```python
from build123d import *

# Parameters (mm, degrees)
SKETCH1_R               = 90
BOSS_EXTRUDE1_DEPTH     = 2
CUT_EXTRUDE2_DEPTH      = 128.294933128
SKETCH9_R               = 1.75
CUT_EXTRUDE7_DEPTH      = 128.294933128
CUT_EXTRUDE8_DEPTH      = 128.294933128
CUT_EXTRUDE8_DEPTH_BACK = 128.294933128
CHAMFER3_SIZE           = 1
SKETCH17_R              = 6
CUT_EXTRUDE9_DEPTH      = 99.491613961


with BuildPart() as part:
    # Sketch1 → Boss-Extrude1 (new body)
    with BuildSketch(Plane(origin=(0, 0, 0), x_dir=(1, 0, 0), z_dir=(0, 1, 0))):
        with Locations(Location((0, 0, 0), (0, 0, 270))):
            Circle(SKETCH1_R)
    extrude(amount=BOSS_EXTRUDE1_DEPTH)

    # Sketch4 → Cut-Extrude2 (cut, through all)
    with BuildSketch(Plane(origin=(0, 2, 0), x_dir=(1, 0, 0), z_dir=(0, 1, 0))):
        with BuildLine():
            Line((-42.5, 79.333158263), (-42.5, 69.333158263))
            ThreePointArc((-42.5, 69.333158263), (0, 55), (42.5, 69.333158263))
            Line((42.5, 69.333158263), (42.5, 79.333158263))
            Line((42.5, 79.333158263), (42.5, 105.809765059))
            Line((42.5, 105.809765059), (-42.5, 105.809765059))
            Line((-42.5, 105.809765059), (-42.5, 79.333158263))
        make_face()
    extrude(amount=-CUT_EXTRUDE2_DEPTH, mode=Mode.SUBTRACT)

    # Sketch9 → Cut-Extrude7 (cut, through all)
    with BuildSketch(Plane(origin=(0, 2, 0), x_dir=(1, 0, 0), z_dir=(0, 1, 0))):
        with Locations(Location((-49.706440821, 70.180266036, 0), (0, 0, 270))):
            Circle(SKETCH9_R)
    cut_extrude7 = extrude(amount=-CUT_EXTRUDE7_DEPTH, mode=Mode.SUBTRACT)

    # Mirror1: Cut-Extrude7 across plane
    add(cut_extrude7.mirror(Plane(origin=(0, 0, 0), x_dir=(0, 0, 1), z_dir=(1, 0, 0))), mode=Mode.SUBTRACT)

    # Sketch10 → Cut-Extrude8 (cut, two sides)
    with BuildSketch(Plane.XZ) as cut_extrude8_sk:
        Polygon((349.590781265, -403.844847198), (57.81736756, -68.972110366), (50, -60), (25, -35), (-25, -35), (-50, -60), (-57.81736756, -68.972110366), (-349.590781265, -403.844847198), (-349.590781265, 484.460223862), (349.590781265, 484.460223862), align=None)
    extrude(amount=CUT_EXTRUDE8_DEPTH, mode=Mode.SUBTRACT)
    extrude(cut_extrude8_sk.sketch, amount=-CUT_EXTRUDE8_DEPTH_BACK, mode=Mode.SUBTRACT)

    # Sketch15 for Loft1 → Loft1 section 0
    with BuildSketch(Plane(origin=(0, -6, 0), x_dir=(1, 0, 0), z_dir=(0, 1, 0))):
        with BuildLine():
            Line((-42.5, 69.333158263), (-42.5, 79.333158263))
            # circular arc as an exact rational Bezier (weights 1, cos(half-angle), 1)
            Bezier((-42.5, 79.333158263), (0, 57.45059928), (42.5, 79.333158263), weights=[1, 0.889071458, 1])
            Line((42.5, 79.333158263), (42.5, 69.333158263))
            Bezier((42.5, 69.333158263), (0, 36.987960736), (-42.5, 69.333158263), weights=[1, 0.795754331, 1])
        make_face()
    # Sketch16 for Loft1 → Loft1 section 1
    with BuildSketch(Plane.XZ):
        with BuildLine():
            Line((-45.948502669, -63.851980058), (-42.5, -69.333158263))
            Bezier((-42.5, -69.333158263), (0, -36.987960736), (42.5, -69.333158263), weights=[1, 0.795754331, 1])
            Line((42.5, -69.333158263), (44.152042302, -63.851980058))
            Bezier((44.152042302, -63.851980058), (-0.898230184, -19.650095816), (-45.948502669, -63.851980058), weights=[1, 0.713795953, 1])
        make_face()
    loft()

    # Chamfer3
    chamfer3_edges = [part.edges().sort_by_distance(p)[0] for p in [
        (0, 2, -55),
    ]]
    chamfer(chamfer3_edges, length=CHAMFER3_SIZE)

    # Sketch17 → Cut-Extrude9 (cut, through all)
    with BuildSketch(Plane(origin=(0, 2, 0), x_dir=(1, 0, 0), z_dir=(0, 1, 0))):
        with Locations(Location((2.697741472, 47.316027374, 0), (0, 0, 270))):
            Circle(SKETCH17_R)
        with Locations(Location((27.628576658, 52.274065286, 0), (0, 0, 270))):
            Circle(SKETCH17_R)
        with Locations(Location((-29.151926102, 52.274065286, 0), (0, 0, 270))):
            Circle(SKETCH17_R)
    extrude(amount=-CUT_EXTRUDE9_DEPTH, mode=Mode.SUBTRACT)


solid = part.part
```
Design review of the part built by this model. Coordinates are the model's own, in mm. A direction names the side the tool comes from. Give positions to 0.01 mm unless a question says otherwise; leave off trailing zeros. Order: outer loops, then holes, each group sorted by start corner. A loop starts at its lowest first (then second) coordinate and runs counter-clockwise, first axis right, second up. Notation, with made-up numbers: (8.25, 82.25) - (28.25, 82.25) arc R20 ccw to (28.25, 115.25) - close; hole circle Ø9 at (-27.5, 38.25). An arc over 180 degrees is marked (long way). Use a Markdown table: item, result. Add a question column.
(1) Mouldability with a two-part tool opening along Z and no side actions: class faces 1 (the face through (0, 1, -35)), 2 (the face through (-0.6, 1.2, -54.8)), 3 (the face through (-28.89, -0.43, -58.27)) as +Z half, -Z half, draft (parallel to the pull), parting line (faces both ways), or undercut.
(2) Add section A-A on z = -57. Give the number of separate pieces and of enclosed holes in the cut face, then the cut area to 3 significant figures.
(3) Clearance check with flat-ended pins moving along their axes: P1, Ø5, axis at x = -25, z = -55, coming from the -Y side; P2, Ø2, axis at x = -14.5, y = -5, coming from the +Z side; P3, Ø12, axis at x = 46, z = -53.5, coming from the -Y side; P4, Ø15.5, axis at x = 2.7, z = -47.32, coming from the +Y side. State where each tip first meets the part, or that it passes through.
(4) Add section B-B on z = -40. Give the boundary of the cut face in (x, y).
(5) Machinability: for faces 4 (the face through (2.96, -0.64, -53.31)), 5 (the face through (-0.639, 0.507, -55.003)), which of the approach directions +Z, -Z, +X, -X, +Y, -Y give a long, thin tool a straight path to every point of the face, cutting with its end or side? Answer none if there is none.
(6) Wall thickness on probe 1 along Y at (x, z) = (-49, -64); probe 2 along X at (y, z) = (1.75, -66); probe 3 along Z at (x, y) = (-50, 0.25): over which ranges is each line inside the solid? List them lowest first. Write a range as [from, to].
Report:
| question | item | result |
|---|---|---|
| 1 | face 1 | +Z half |
| 1 | face 2 | -Z half |
| 1 | face 3 | undercut |
| 2 | separate pieces | 3 |
| 2 | enclosed holes | 0 |
| 2 | area | 363 mm² |
| 3 | P1 | stops at y = -4.76 |
| 3 | P2 | stops at z = -53.31 |
| 3 | P3 | stops at y = 0 |
| 3 | P4 | stops at y = 2 |
| 4 | outline | (-30, 0) - (30, 0) - (30, 2) - (-30, 2) - close |
| 5 | face 4 | +Y, -Y |
| 5 | face 5 | -Z, +Y |
| 6 | probe 1 | y = [0, 2] |
| 6 | probe 2 | x = [-55.23, -39.1], [39.1, 55.23] |
| 6 | probe 3 | z = [-74.83, -71.91], [-68.46, -60] |
